from build123d import *

# Parameters (mm, degrees)
RESSALTO_EXTRUS_O1_DEPTH = 9.5
FILETE1_R                = 0.2
ESBO_O3_R                = 1.0922
CORTE_EXTRUS_O1_DEPTH    = 4.76
ESBO_O2_R                = 1.0922
CORTE_EXTRUS_O2_DEPTH    = 10.5


with BuildPart() as part:
    # Esboço1 → Ressalto-extrusão1 (new body)
    with BuildSketch(Plane(origin=(0, 0, 0), x_dir=(1, 0, 0), z_dir=(0, 1, 0))):
        Polygon((2.748187281, 0), (1.374093641, 2.38), (-1.374093641, 2.38), (-2.748187281, 0), (-1.374093641, -2.38), (1.374093641, -2.38), align=None)
    extrude(amount=RESSALTO_EXTRUS_O1_DEPTH)

    # Filete1
    filete1_edges = [part.edges().sort_by_distance(p)[0] for p in [
        (0, 9.5, -2.38),
        (-2.061140461, 9.5, -1.19),
        (-2.061140461, 9.5, 1.19),
        (0, 9.5, 2.38),
        (2.061140461, 9.5, 1.19),
        (0, 0, 2.38),
        (-2.061140461, 0, 1.19),
        (-2.061140461, 0, -1.19),
        (2.061140461, 9.5, -1.19),
        (0, 0, -2.38),
        (2.061140461, 0, -1.19),
        (2.061140461, 0, 1.19),
    ]]
    fillet(filete1_edges, radius=FILETE1_R)

    # Esboço3 → Corte-extrusão1 (cut)
    with BuildSketch(Plane(origin=(0, 9.5, 0), x_dir=(1, 0, 0), z_dir=(0, 1, 0))):
        Circle(ESBO_O3_R)
    extrude(amount=-CORTE_EXTRUS_O1_DEPTH, mode=Mode.SUBTRACT)

    # Esboço2 → Corte-extrusão2 (cut, through all)
    with BuildSketch(Plane.XZ):
        Circle(ESBO_O2_R)
    extrude(amount=-CORTE_EXTRUS_O2_DEPTH, mode=Mode.SUBTRACT)


solid = part.part
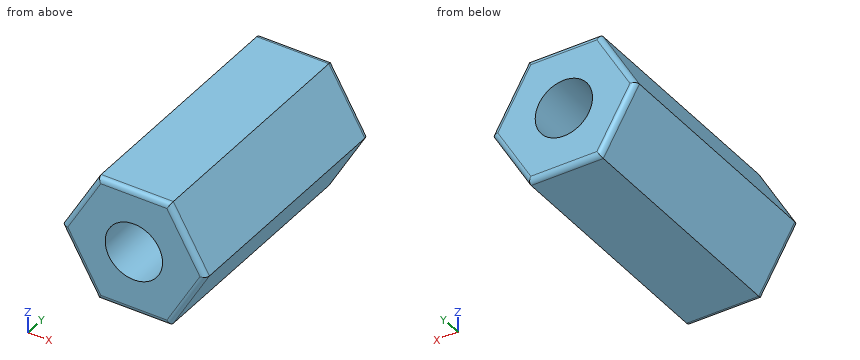
Design review of the part built by this model. Coordinates are the model's own, in mm. Give positions to 0.01 mm unless a question says otherwise; leave off trailing zeros. Write each loop counter-clockwise with the first axis right and the second up, starting at its lowest first coordinate (ties: lowest second). Pieces come first, ordered by that corner, then holes. Notation, with made-up numbers: M 54.25,5.5 L 80.25,5.5 A19 ccw 80.25,20.5 Z; hole C 78.25,38.25 d6. An arc over 180 degrees is marked long. Return JSON: item names as keys, results as strings. Group by question number.
Item 1: Clearance check with a flat-ended pin moving along its axis: pin 1 Ø1.5 at (y, z) = (5, -1.5) entering from +X. State where the tip first meets the part, or that it passes through.
Item 2: Wall thickness on line 1 along Z through (x, y) = (0, 2); line 2 along Z through (x, y) = (0.5, 3.5); line 3 along X through (y, z) = (2.5, -0.7): over which ranges is each line inside the solid? List them lowest first.
Item 3: Take a section at B-B (y = 2.5). Give the boundary of the cut face in (x, z).
Item 4: Take a section at A-A (x = 0). Give the boundary of the cut face in (y, z), plus the area to 3 significant figures.
Item 5: Take a section at C-C (x = -0.95). Give the boundary of the cut face in (y, z).
Return value:
{
 "1": {"pin 1": "stops at x = 2.32"},
 "2": {"line 1": "z = -2.38 to -1.09, 1.09 to 2.38", "line 2": "z = -2.38 to -0.97, 0.97 to 2.38", "line 3": "x = -2.34 to -0.84, 0.84 to 2.34"},
 "3": {"outline": "M -2.75,0 L -1.37,-2.38 L 1.37,-2.38 L 2.75,0 L 1.37,2.38 L -1.37,2.38 Z; hole C 0,0 d2.18"},
 "4": {"outline": "M 0,-2.18 A0.2 ccw 0.2,-2.38 L 9.3,-2.38 A0.2 ccw 9.5,-2.18 L 9.5,-1.09 L 0,-1.09 Z; M 0,1.09 L 9.5,1.09 L 9.5,2.18 A0.2 ccw 9.3,2.38 L 0.2,2.38 A0.2 ccw 0,2.18 Z", "area": "24.4 mm2"},
 "5": {"outline": "M 0,-2.18 A0.2 ccw 0.2,-2.38 L 9.3,-2.38 A0.2 ccw 9.5,-2.18 L 9.5,-0.54 L 0,-0.54 Z; M 0,0.54 L 9.5,0.54 L 9.5,2.18 A0.2 ccw 9.3,2.38 L 0.2,2.38 A0.2 ccw 0,2.18 Z"}
}
